Input: dimensioned drawing with shaded views. Units: mm. Origin: part minimum x, y, z. A direction names the side the tool comes from. Give positions to 0.01 mm unless a question says otherwise; leave off trailing zeros. Order: outer loops, then holes, each group sorted by start corner. A loop starts at its lowest first (then second) coordinate and runs counter-clockwise, first axis right, second up. Notation, with made-up numbers: (9.5, 59.5) - (61.5, 59.5) arc R3 ccw to (61.5, 63.5) - close; hole circle Ø10 at (12, -3). An arc over 180 degrees is marked (long way). Use a Markdown table: item, result.
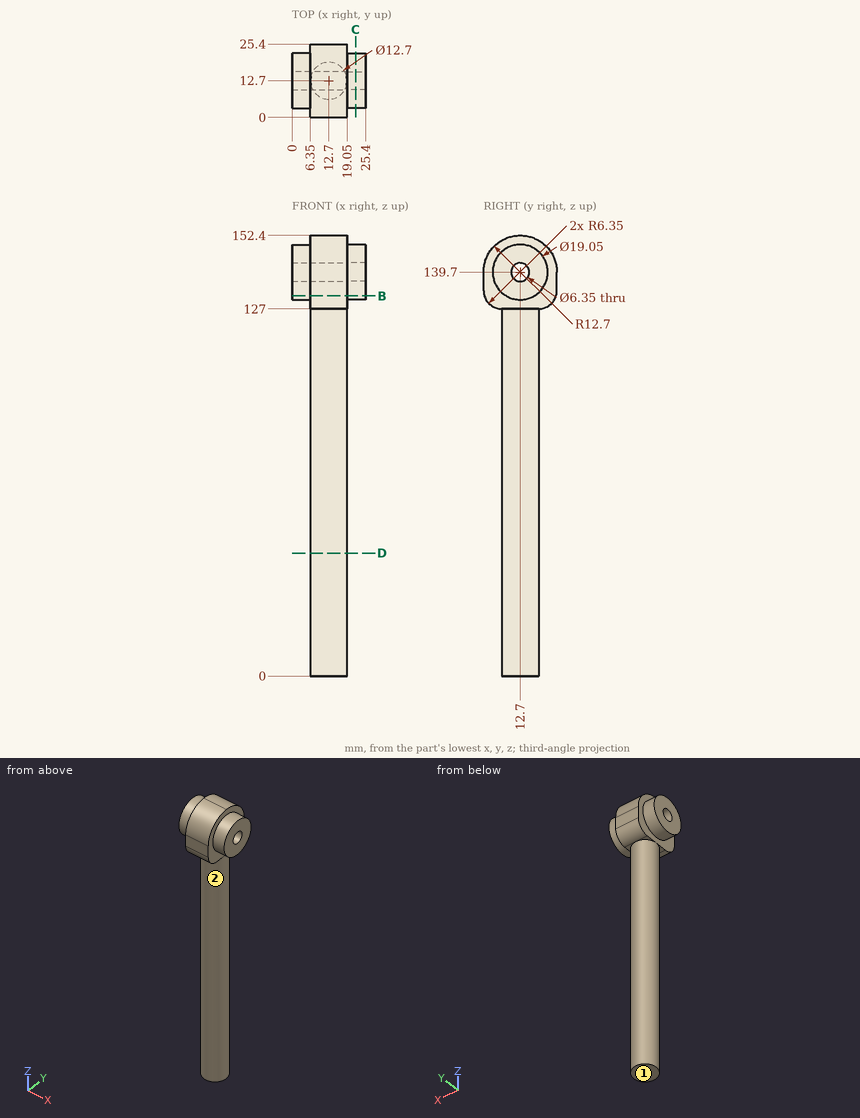
1. Material intervals for line 1 along Y through (x, z) = (9, 139.7) (3 decimals); line 2 along Z through (x, y) = (4, 12.7) (3 decimals); line 3 along Z through (x, y) = (10.5, 12.7) (3 decimals), sorted ascending.
Response:
| item | result |
|---|---|
| line 1 | y = 0 to 9.525, 15.875 to 25.4 |
| line 2 | z = 130.175 to 136.525, 142.875 to 149.225 |
| line 3 | z = 0 to 136.525, 142.875 to 152.4 |
2. Set-up query: the marked faces 1 and 2. Return all of +Z, -Z, +X, -X, +Y, -Y with unobstructed straight access to the full face (end or side cutting, diameter ignored); none if empty.
Response:
| item | result |
|---|---|
| face 1 | -Z, +X, -X, +Y, -Y |
| face 2 | -Z |
3. Pin query (flat end, axial travel): pin 1 (1 mm diameter, centred on x = 21.5, y = 20.5, fed in from -Z); pin 2 (5 mm diameter, centred on x = 14, z = 49, fed in from +Y); pin 3 (2 mm diameter, centred on x = 8.5, z = 23.5, fed in from -Y); pin 4 (4 mm diameter, centred on y = 12.7, z = 139.7, fed in from +X). Return the tip coordinate at first contact, or that it passes through.
Response:
| item | result |
|---|---|
| pin 1 | stops at z = 133.58 |
| pin 2 | stops at y = 19.05 |
| pin 3 | stops at y = 7.22 |
| pin 4 | passes through |
4. Section query C-C (x = 22). Return loops of the section in (y, z) (3 decimals).
Response:
| item | result |
|---|---|
| outline | circle Ø19.05 at (12.7, 139.7); hole circle Ø6.35 at (12.7, 139.7) |
5. Section query D-D (z = 42.5). Return loops of the section in (x, y).
Response:
| item | result |
|---|---|
| outline | circle Ø12.7 at (12.7, 12.7) |
6. Section query B-B (z = 131.5). Return loops of the section in (x, y), then the cut area to 3 significant figures.
Response:
| item | result |
|---|---|
| outline | (0, 7.85) - (6.35, 7.85) - (6.35, 0.28) - (19.05, 0.28) - (19.05, 7.85) - (25.4, 7.85) - (25.4, 17.55) - (19.05, 17.55) - (19.05, 25.12) - (6.35, 25.12) - (6.35, 17.55) - (0, 17.55) - close |
| area | 439 mm^2 |
